Read the model definition and answer for the solid it produces. Units are mm, in the model's axes. Face numbers are marked on the shaded views. A direction names the side the tool comes from. Coordinates: 2 decimals unless noted, no trailing zeros. Order: outer loops, then holes, each group sorted by start corner. A loop starts at its lowest first (then second) coordinate and runs counter-clockwise, first axis right, second up. Notation, with made-up numbers: (35, -26.75) -> (88, -26.75) arc R20 ccw to (88, -4.75) -> close; hole circle Ø2 at (-35.5, 68.5). An arc over 180 degrees is marked (long way). Use CSV: the item, a comma, the result in double quotes.
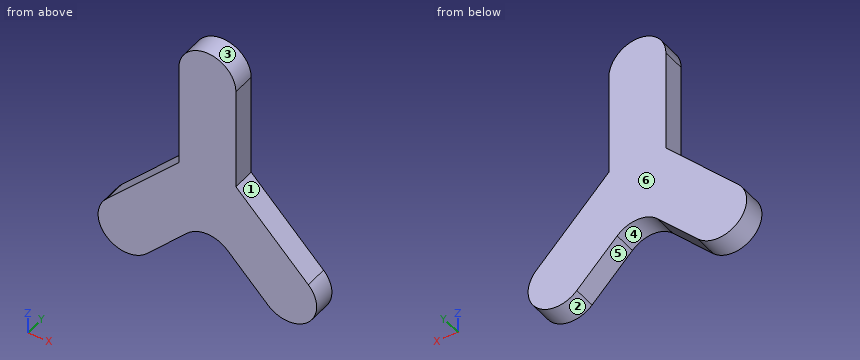
```python
from build123d import *

# Parameters (mm, degrees)
BOSS_EXTRUDE1_DEPTH = 2


with BuildPart() as part:
    # Sketch1 → Boss-Extrude1 (new body)
    with BuildSketch(Plane(origin=(0, 0, 0), x_dir=(1, 0, 0), z_dir=(0, 1, 0))):
        with BuildLine():
            Line((2.5, -10), (2.5, -1.035533906))
            Line((2.5, -1.035533906), (8.838834765, 5.303300859))
            ThreePointArc((8.838834765, 5.303300859), (8.838834765, 8.838834765), (5.303300859, 8.838834765))
            Line((5.303300859, 8.838834765), (1.767766953, 5.303300859))
            ThreePointArc((1.767766953, 5.303300859), (0, 4.571067812), (-1.767766953, 5.303300859))
            Line((-1.767766953, 5.303300859), (-5.303300859, 8.838834765))
            ThreePointArc((-5.303300859, 8.838834765), (-8.838834765, 8.838834765), (-8.838834765, 5.303300859))
            Line((-8.838834765, 5.303300859), (-2.5, -1.035533906))
            Line((-2.5, -1.035533906), (-2.5, -10))
            ThreePointArc((-2.5, -10), (0, -12.5), (2.5, -10))
        make_face()
    extrude(amount=BOSS_EXTRUDE1_DEPTH)


solid = part.part
```
Item 1: Find section A-A, the plane y = 1.6. Give the vertices of the cut face in (x, z).
Return value:
outline,"(-8.84, -5.3) arc R2.5 ccw to (-5.3, -8.84) -> (-1.77, -5.3) arc R2.5 cw to (1.77, -5.3) -> (5.3, -8.84) arc R2.5 ccw to (8.84, -5.3) -> (2.5, 1.04) -> (2.5, 10) arc R2.5 ccw to (-2.5, 10) -> (-2.5, 1.04) -> close"
Item 2: Find section B-B, the plane z = 7. Give the vertices of the cut face in (x, y), then the cut area to 3 significant figures.
Return value:
outline,"(-2.5, 0) -> (2.5, 0) -> (2.5, 2) -> (-2.5, 2) -> close"
area,"10.0 mm^2"
Item 3: Straight lines are drawn through the part: line 1 along X through (y, z) = (1.8, 4); line 2 along X through (y, z) = (1.95, -6.5); line 3 along X through (y, z) = (1.4, -5). For each, find the intervals that lie inside material, in ascending order.
Return value:
line 1,"x = -2.5 to 2.5"
line 2,"x = -9.5 to -2.96, 2.96 to 9.5"
line 3,"x = -8.54 to -1.4, 1.4 to 8.54"
Item 4: Find section C-C, the plane x = 6.25. Give the vertices of the cut face in (y, z).
Return value:
outline,"(0, -9.43) -> (2, -9.43) -> (2, -2.71) -> (0, -2.71) -> close"
Item 5: The mould has two halves that part along X. Classify the marked faces 1, 2, 3 and 4: +X half, -X half, draft (parallel to the pull), parting line (faces both ways), or undercut.
Return value:
face 1,"+X half"
face 2,"undercut"
face 3,"parting line"
face 4,"undercut"
Item 6: Each of these flat-tipped pins is pushed along its axis until it touches: P1, Ø1, axis at y = 1.5, z = 6.5, coming from the -X side; P2, Ø1, axis at y = 1.5, z = 3, coming from the +X side. Where does it stop, or does it pass through?
Return value:
P1,"stops at x = -2.5"
P2,"stops at x = 2.5"
Item 7: A tool of negligible diameter and unlimited length cuts with its end or side. For the marked faces 5 and 6, from which of +Z, -Z, +X, -X, +Y, -Y can it reach the whole face along a straight path? Write none if from no direction.
Return value:
face 5,"-Z, +Y, -Y"
face 6,"+Z, -Z, +X, -X, +Y"
